Read the model definition and answer for the solid it produces. Units are mm, in the model's axes. A direction names the side the tool comes from. Round coordinates to 2 decimals unless told otherwise and drop trailing zeros. Write each loop counter-clockwise with the first axis right and the second up, starting at its lowest first coordinate (ties: lowest second). Pieces come first, ordered by that corner, then holes. Notation, with made-up numbers: (44, -32.5) -> (67, -32.5) arc R26 cw to (67, -3.5) -> close; hole circle Ø9 at (-32, 48). An arc over 180 degrees is marked (long way). Return JSON: item names as keys, results as strings. Group by question number.
(1) A cutting plane is placed at C-C on z = 25. Give the vertices of the cut face in (x, y), then the cut area to 3 significant figures.
(2) For faces 1 (the flat face through (26.2, -5.8, 11.7)), 2 (the flat face through (26, 6, 52)), 3 (the flat face through (26.2, 5.8, 11.7)), 4 (the flat face through (28.7, -5.7, 48.2)), determine the directions among +Z, -Z, +X, -X, +Y, -Y from which every point of the face is accessible in a straight line to the end or side of a thin tool.
(3) Straight lines are drawn through the part: line 1 (Z direction, x = 45.5, y = -5.25); line 2 (Z direction, x = 8, y = -0.5); line 3 (X direction, y = -2.75, z = 39). For each, find the intervals that lie inside material, in ascending order.
(4) A cutting plane is placed at D-D on y = 6.5. Give the vertices of the cut face in (x, z).
(5) The mould has two halves that part along Z. Classify faces 5 (the cylindrical face through (-7.5, 0.16, 2.46)), 6 (the flat face through (38.5, -3.4, 55)), 7 (the flat face through (26, 4, 31)): released by +Z, released by -Z, zero draft, split by the parting line, or undercut.
(6) A cutting plane is placed at B-B on y = 0.75. State how many separate pieces and enclosed holes the cut face has, then the cut area to 3 significant figures.
(7) Given pin 1 (7.5 mm diameter, centred on x = 12, y = -3, fed in from +Z); pin 2 (3 mm diameter, centred on x = 0.5, y = 2, fed in from -Z); pin 3 (2 mm diameter, centred on x = 27.5, z = 33, fed in from -Y); pin 4 (4 mm diameter, centred on y = 0, z = 24.27, fed in from +X), each flat-ended and moving along its own axis, determine where each tip first touches the part or whether it passes through.
(8) A cutting plane is placed at A-A on x = 4. Give the vertices of the cut face in (y, z).
```python
from build123d import *

# Parameters (mm, degrees)
SKETCH1_R           = 7.5
SKETCH1_R_2         = 5
BOSS_EXTRUDE1_DEPTH = 5
SKETCH2_W           = 5
SKETCH2_H           = 15
BOSS_EXTRUDE2_DEPTH = 55
SKETCH3_W           = 5
SKETCH3_H           = 15
BOSS_EXTRUDE3_DEPTH = 20
SKETCH4_R           = 5
CUT_EXTRUDE1_DEPTH  = 15
FILLET1_R           = 7.5
CHAMFER1_SIZE       = 5
CUT_EXTRUDE2_DEPTH  = 5
CHAMFER2_SIZE       = 1.5
CHAMFER3_SIZE       = 2.5
CHAMFER4_SIZE       = 2.5
SKETCH6_R           = 1.75
CUT_EXTRUDE3_DEPTH  = 10


with BuildPart() as part:
    # Sketch1 → Boss-Extrude1 (new body)
    # profile 1 of 2: a face of its own
    with BuildSketch(Plane.XY):
        Circle(SKETCH1_R)
        Circle(SKETCH1_R_2, mode=Mode.SUBTRACT)
    # profile 2 of 2: a face of its own
    with BuildSketch(Plane.XY):
        with BuildLine():
            Line((30, 7.5), (0, 7.5))
            ThreePointArc((0, 7.5), (5.303300859, 5.303300859), (7.5, 0))
            ThreePointArc((7.5, 0), (5.303300859, -5.303300859), (0, -7.5))
            Line((0, -7.5), (30, -7.5))
            Line((30, -7.5), (30, 7.5))
        make_face()
    extrude(amount=BOSS_EXTRUDE1_DEPTH)

    # Sketch2 → Boss-Extrude2 (add)
    with BuildSketch(Plane.XY.offset(5)):
        with Locations((27.5, 0)):
            Rectangle(SKETCH2_W, SKETCH2_H)
    extrude(amount=BOSS_EXTRUDE2_DEPTH)

    # Sketch3 → Boss-Extrude3 (add)
    with BuildSketch(Plane(origin=(30, 0, 0), x_dir=(0, 0, -1), z_dir=(1, 0, 0))):
        with Locations((-57.5, 0)):
            Rectangle(SKETCH3_W, SKETCH3_H)
    extrude(amount=BOSS_EXTRUDE3_DEPTH)

    # Sketch4 → Cut-Extrude1 (cut)
    with BuildSketch(Plane(origin=(0, 0, 55), x_dir=(-1, 0, 0), z_dir=(0, 0, -1))):
        with Locations(Location((-42.5, 0, 0), (0, 0, 90))):
            Circle(SKETCH4_R)
    extrude(amount=-CUT_EXTRUDE1_DEPTH, mode=Mode.SUBTRACT)

    # Fillet1
    fillet1_edges = [part.edges().sort_by_distance(p)[0] for p in [
        (50, -7.5, 57.5),
        (50, 7.5, 57.5),
    ]]
    fillet(fillet1_edges, radius=FILLET1_R - 0.0001)  # a hair under: the kernel refuses the full size

    # Chamfer1
    chamfer1_edges = [part.edges().sort_by_distance(p)[0] for p in [
        (25, 0, 5),
        (25, 0, 60),
        (30, 0, 55),
        (30, 0, 0),
    ]]
    chamfer(chamfer1_edges, length=CHAMFER1_SIZE)

    # Sketch5 → Cut-Extrude2 (cut)
    with BuildSketch(Plane.ZY.offset(-25)):
        Polygon((10, -7.5), (13, -4.5), (47, -4.5), (50, -7.5), align=None)
        Polygon((50, 7.5), (10, 7.5), (13, 4.5), (47, 4.5), align=None)
    extrude(amount=-CUT_EXTRUDE2_DEPTH, mode=Mode.SUBTRACT)

    # Chamfer2
    chamfer2_edges = [part.edges().sort_by_distance(p)[0] for p in [
        (25, -4.5, 30),
        (30, 4.5, 30),
        (25, 4.5, 30),
        (30, -4.5, 30),
    ]]
    chamfer(chamfer2_edges, length=CHAMFER2_SIZE)

    # Chamfer3
    chamfer3_edges = [part.edges().sort_by_distance(p)[0] for p in [
        (30, 5.25, 12.25),
        (25, 5.25, 47.75),
        (25, 7.5, 52.5),
        (27.5, 7.5, 57.5),
        (27.5, 7.5, 2.5),
        (25, -7.5, 52.5),
        (27.5, -7.5, 57.5),
        (27.5, -7.5, 2.5),
        (30, 7.5, 7.5),
        (30, -7.5, 7.5),
        (30, -5.25, 12.25),
        (25, -5.25, 47.75),
    ]]
    chamfer(chamfer3_edges, length=CHAMFER3_SIZE)

    # Chamfer4
    chamfer4_edges = [part.edges().sort_by_distance(p)[0] for p in [
        (22.5, -7.5, 7.5),
        (22.5, 7.5, 7.5),
        (32.5, 7.5, 52.5),
        (32.5, -7.5, 52.5),
    ]]
    chamfer(chamfer4_edges, length=CHAMFER4_SIZE)

    # Sketch6 → Cut-Extrude3 (cut)
    with BuildSketch(Plane.ZY.offset(-25)):
        with Locations((31.767766953, 0)):
            Circle(SKETCH6_R)
        with Locations((39.267766953, 0)):
            Circle(SKETCH6_R)
        with Locations((24.267766953, 0)):
            Circle(SKETCH6_R)
    extrude(amount=-CUT_EXTRUDE3_DEPTH, mode=Mode.SUBTRACT)


solid = part.part
```
Checks:
{
 "1": {"outline": "(25, -3) -> (26.5, -4.5) -> (28.5, -4.5) -> (30, -3) -> (30, -1.59) -> (25, -1.59) -> close; (25, 1.59) -> (30, 1.59) -> (30, 3) -> (28.5, 4.5) -> (26.5, 4.5) -> (25, 3) -> close", "area": "24.6 mm^2"},
 "2": {"face 1": "-X, -Y", "face 2": "+Z, -X, +Y", "face 3": "-X, +Y", "face 4": "+X, -Y"},
 "3": {"line 1": "z = 55 to 60", "line 2": "z = 0 to 5", "line 3": "x = 25 to 30"},
 "4": {"outline": "(-3.74, 0) -> (22.88, 0) -> (28.5, 5.62) -> (28.5, 9.59) -> (27.5, 11) -> (25, 11) -> (25, 7.88) -> (22.12, 5) -> (-3.74, 5) -> close; (26.5, 50.41) -> (27.5, 49) -> (30, 49) -> (30, 52.12) -> (32.88, 55) -> (46.24, 55) -> (46.24, 60) -> (32.12, 60) -> (26.5, 54.38) -> close"},
 "5": {"face 5": "zero draft", "face 6": "released by -Z", "face 7": "undercut"},
 "6": {"separate pieces": "6", "enclosed holes": "0", "area": "416 mm^2"},
 "7": {"pin 1": "stops at z = 5", "pin 2": "passes through", "pin 3": "stops at y = -4.5", "pin 4": "stops at x = 30"},
 "8": {"outline": "(-7.5, 0) -> (-3, 0) -> (-3, 5) -> (-7.5, 5) -> close; (3, 0) -> (7.5, 0) -> (7.5, 5) -> (3, 5) -> close"}
}
